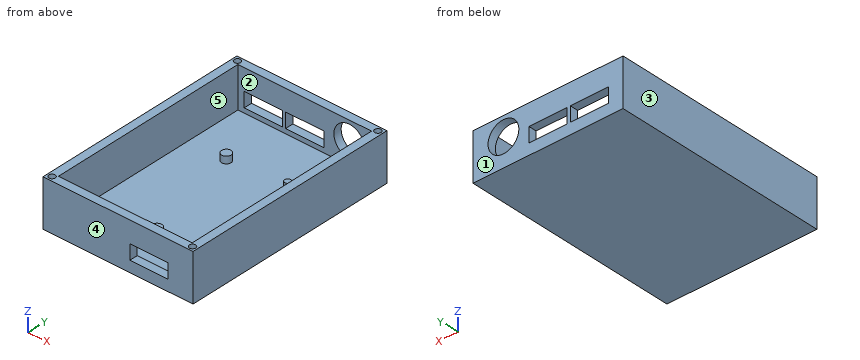
from build123d import *

# Parameters (mm, degrees)
SKETCH1_R             = 2.236067977
BOSS_EXTRUDE1_DEPTH   = 3.25
SKETCH1_R_2           = 1.414213562
BOSS_EXTRUDE1_2_DEPTH = 3.25
BOSS_EXTRUDE1_3_DEPTH = 3.25
SKETCH1_21_W          = 70.681980515
SKETCH1_21_H          = 102.181980515
BOSS_EXTRUDE2_DEPTH   = 3
SKETCH1_23_W          = 70.681980515
SKETCH1_23_H          = 102.181980515
SKETCH1_23_R          = 1.5
SKETCH1_23_W_2        = 63
SKETCH1_23_H_2        = 94.5
BOSS_EXTRUDE4_DEPTH   = 19.25
SKETCH3_R             = 7.25
SKETCH3_W             = 18
SKETCH3_H             = 7
CUT_EXTRUDE1_DEPTH    = 3.84099
SKETCH4_W             = 18
SKETCH4_H             = 7
CUT_EXTRUDE2_DEPTH    = 3.84099


with BuildPart() as part:
    # Sketch1 → Boss-Extrude1 (new body)
    with BuildSketch(Plane.XY):
        with Locations((22, 72)):
            Circle(SKETCH1_R)
    extrude(amount=BOSS_EXTRUDE1_DEPTH)



with BuildPart() as body_2:
    # Sketch1 → Boss-Extrude1 2 (new body)
    with BuildSketch(Plane.XY):
        with Locations((50, 73)):
            Circle(SKETCH1_R_2)
    extrude(amount=BOSS_EXTRUDE1_2_DEPTH)


with BuildPart() as body_3:
    # Sketch1 → Boss-Extrude1 3 (new body)
    with BuildSketch(Plane.XY):
        with Locations((35, 21)):
            Circle(SKETCH1_R)
    extrude(amount=BOSS_EXTRUDE1_3_DEPTH)


with BuildPart() as part_1:
    add(part.part)

    add(body_2.part)  # Boss-Extrude2 merges body 2

    add(body_3.part)  # Boss-Extrude2 merges body 3
    # Sketch1<21> → Boss-Extrude2 (add)
    with BuildSketch(Plane.XY):
        with Locations((35.340990258, 51.090990258)):
            Rectangle(SKETCH1_21_W, SKETCH1_21_H)
    extrude(amount=-BOSS_EXTRUDE2_DEPTH)

    # Sketch1<23> → Boss-Extrude4 (add)
    with BuildSketch(Plane.XY):
        with Locations((35.340990258, 51.090990258)):
            Rectangle(SKETCH1_23_W, SKETCH1_23_H)
        with BuildLine():
            ThreePointArc((3.75, 2.25), (0.864180701, 1.675974851), (3.310660172, 3.310660172))
            ThreePointArc((3.310660172, 3.310660172), (3.635819299, 2.824025149), (3.75, 2.25))
        make_face(mode=Mode.SUBTRACT)
        with Locations((68.431980515, 2.25)):
            Circle(SKETCH1_23_R, mode=Mode.SUBTRACT)
        with Locations((2.25, 99.931980515)):
            Circle(SKETCH1_23_R, mode=Mode.SUBTRACT)
        with Locations((35.340990258, 51.090990258)):
            Rectangle(SKETCH1_23_W_2, SKETCH1_23_H_2, mode=Mode.SUBTRACT)
        with Locations((68.431980515, 99.931980515)):
            Circle(SKETCH1_23_R, mode=Mode.SUBTRACT)
    extrude(amount=BOSS_EXTRUDE4_DEPTH)

    # Sketch3 → Cut-Extrude1 (cut)
    with BuildSketch(Plane.XZ.offset(-98.340990258)):
        with Locations((56.340990258, 10.25)):
            Circle(SKETCH3_R)
        with Locations((15.840990258, 5.75)):
            Rectangle(SKETCH3_W, SKETCH3_H)
        with Locations((35.340990258, 5.75)):
            Rectangle(SKETCH3_W, SKETCH3_H)
    extrude(amount=-CUT_EXTRUDE1_DEPTH, mode=Mode.SUBTRACT)

    # Sketch4 → Cut-Extrude2 (cut)
    with BuildSketch(Plane.XZ):
        with Locations((49.931980515, 5.75)):
            Rectangle(SKETCH4_W, SKETCH4_H)
    extrude(amount=-CUT_EXTRUDE2_DEPTH, mode=Mode.SUBTRACT)


solid = part_1.part
For this review, take the finished solid that the model builds, in its own axes (mm). Face numbers are marked on the shaded views. A direction names the side the tool comes from. Round coordinates to 2 decimals unless told otherwise and drop trailing zeros. Order: outer loops, then holes, each group sorted by start corner. A loop starts at its lowest first (then second) coordinate and runs counter-clockwise, first axis right, second up. Notation, with made-up numbers: (41.5, 43) -> (78.5, 43) arc R21 cw to (78.5, 72) -> close; hole circle Ø9 at (-34, 53.25). An arc over 180 degrees is marked (long way). Write item = value, one per line. Start each with the question number.
1) Take a section at C-C on x = 2.25. State the section outline as (y, z) points, plus the area to 3 significant figures.
2) Insertion check: pin 1 (3.5 mm diameter, centred on x = 68, y = 3, fed in from +Z); pin 2 (1.5 mm diameter, centred on x = 14.5, y = 76, fed in from +Z); pin 3 (3.5 mm diameter, centred on x = 21.5, y = 72, fed in from +Z); pin 4 (3 mm diameter, centred on x = 59.5, z = 9.5, fed in from +Y). Each pin has a flat end and moves straight along its axis. Give the tip position at first contact, or say it passes through.
3) Take a section at D-D on y = 21. State the section outline as (x, z) points.
4) The part is to be moulded in two halves that separate along X. For the marked faces 1, 2 and 3, say which applies: +X half, -X half, draft (parallel to the pull), parting line (faces both ways), or undercut.
5) To check wall thickness, follow line 1 (Y direction, x = 2.25, z = 11.5); line 2 (X direction, y = 86, z = 11); line 3 (Y direction, x = 46.5, z = 12.5). State the ranges of each line that lie inside material, in increasing order. Write a range as from..to.
6) Take a section at B-B on z = 8. State the section outline as (x, y) points, plus the area to 3 significant figures.
7) Take a section at A-A on x = 22. State the section outline as (y, z) points.
8) Tool access review of the marked faces 4 and 5: name each direction out of +Z, -Z, +X, -X, +Y, -Y from which nothing blocks a thin tool from reaching the whole face with its end or side.
Verdict:
q1.outline = (0, -3) -> (102.18, -3) -> (102.18, 19.25) -> (101.43, 19.25) -> (101.43, 0) -> (98.43, 0) -> (98.43, 19.25) -> (3.75, 19.25) -> (3.75, 0) -> (0.75, 0) -> (0.75, 19.25) -> (0, 19.25) -> close
q1.area = 2,160 mm2
q2.pin_1 = 19.25
q2.pin_2 = 0
q2.pin_3 = 3.25
q2.pin_4 = 3.84
q3.outline = (0, -3) -> (70.68, -3) -> (70.68, 19.25) -> (66.84, 19.25) -> (66.84, 0) -> (37.24, 0) -> (37.24, 3.25) -> (32.76, 3.25) -> (32.76, 0) -> (3.84, 0) -> (3.84, 19.25) -> (0, 19.25) -> close
q4.face_1 = draft
q4.face_2 = undercut
q4.face_3 = -X half
q5.line_1 = 0..0.75, 3.75..98.43, 101.43..102.18
q5.line_2 = 0..3.84, 66.84..70.68
q5.line_3 = 0..3.84, 98.34..102.18
q6.outline = (0, 0) -> (40.93, 0) -> (40.93, 3.84) -> (3.84, 3.84) -> (3.84, 98.34) -> (6.84, 98.34) -> (6.84, 102.18) -> (0, 102.18) -> close; (24.84, 98.34) -> (26.34, 98.34) -> (26.34, 102.18) -> (24.84, 102.18) -> close; (44.34, 98.34) -> (49.45, 98.34) -> (49.45, 102.18) -> (44.34, 102.18) -> close; (58.93, 0) -> (70.68, 0) -> (70.68, 102.18) -> (63.23, 102.18) -> (63.23, 98.34) -> (66.84, 98.34) -> (66.84, 3.84) -> (58.93, 3.84) -> close; hole circle Ø3 at (2.25, 2.25); hole circle Ø3 at (2.25, 99.93); hole circle Ø3 at (68.43, 2.25); hole circle Ø3 at (68.43, 99.93)
q6.area = 980 mm2
q7.outline = (0, -3) -> (102.18, -3) -> (102.18, 2.25) -> (98.34, 2.25) -> (98.34, 0) -> (74.24, 0) -> (74.24, 3.25) -> (69.76, 3.25) -> (69.76, 0) -> (3.84, 0) -> (3.84, 19.25) -> (0, 19.25) -> close; (98.34, 9.25) -> (102.18, 9.25) -> (102.18, 19.25) -> (98.34, 19.25) -> close
q8.face_4 = +Z, -Z, +X, -X, -Y
q8.face_5 = +Z
